Source: CAD feature listing. Evaluate the final solid. Frame: model axes, mm. A direction names the side the tool comes from. Give positions to 0.01 mm unless a question says otherwise; leave off trailing zeros. Loops run counter-clockwise (first coordinate to the right, second up) from the corner with the lowest first, then second, coordinate; pieces in that order, holes last.
```python
from build123d import *

# Parameters (mm, degrees)
F0_R     = 25
F1_DEPTH = 6
F2_R     = 21.4280280098
F3_DEPTH = 3
F4_SIZE  = 5
F6_R     = 21.8410066176
F7_DEPTH = 4
F8_R     = 21.2290439381
F9_DEPTH = 25


# Not quite as in the source:
# - a fillet or chamfer that OpenCascade refuses, or shapes differently, is made with other operations: its cross-section is extruded or revolved along the edge and cut away or added


with BuildPart() as f1:
    # F0 (on Top) → F1 (new body)
    with BuildSketch(Plane.XY):
        Circle(F0_R)
    extrude(amount=F1_DEPTH)

    # F2 (on face) → F3 (join)
    with BuildSketch(Plane.XY.offset(6)):
        Circle(F2_R)
    extrude(amount=-F3_DEPTH)

    # F4
    f4_edges = [f1.edges().sort_by_distance(p)[0] for p in [
        (-25, 0, 6),
    ]]
    chamfer(f4_edges, length=F4_SIZE)

    # F5: fillet of radius 5 on 3 edges, made by hand

    # F5_s1 → F5_t2 (revolve, cut)
    with BuildSketch(Plane.XZ):
        with BuildLine():
            ThreePointArc((25, 0), (24.5002551285, 1.2451619378), (23.687395822, 2.312604178))
            Line((23.687395822, 2.312604178), (25, 1))
            Line((25, 1), (25, 0))
        make_face()
    revolve(axis=Axis((0, 0, 1), (0, 0, 1)), mode=Mode.SUBTRACT)

    # F5_s3 → F5_t4 (revolve, cut)
    with BuildSketch(Plane.XZ):
        with BuildLine():
            ThreePointArc((21.4644660941, 4.5355339059), (19.84234935, 5.6193976626), (17.9289321881, 6))
            Line((17.9289321881, 6), (20, 6))
            Line((20, 6), (21.4644660941, 4.5355339059))
        make_face()
    revolve(axis=Axis((0, 0, 6), (0, 0, 1)), mode=Mode.SUBTRACT)

    # F6 (on face) → F7 (join)
    with BuildSketch(Plane(origin=(0, 0, 0), x_dir=(1, 0, 0), z_dir=(0, 0, -1))):
        Circle(F6_R)
    extrude(amount=-F7_DEPTH)

    # F8 (on face) → F9 (join)
    with BuildSketch(Plane(origin=(0, 0, 0), x_dir=(1, 0, 0), z_dir=(0, 0, -1))):
        Circle(F8_R)
    extrude(amount=F9_DEPTH)


solid = f1.part
```
(1) Ray query, line 1 along Z through (x, y) = (-10.5, -15); line 2 along Y through (x, z) = (0.5, -8.5); line 3 along Y through (x, z) = (18.5, -6). Return the intervals inside material, ascending.
A:
line 1: z = -25 to 5.99
line 2: y = -21.22 to 21.22
line 3: y = -10.41 to 10.41
(2) Reachability of faces 1 (the flat face through (0, 0, -25)), 2 (the flat face through (-11.2, -18.4, 0)) from +Z, -Z, +X, -X, +Y, -Y: full face, straight path, thin tool, end or side. Return the list, or none.
A:
face 1: -Z, +X, -X, +Y, -Y
face 2: -Z
(3) Section C-C, the plane z = -1. Return the cut outline in (x, y), then the cut area to 3 significant figures.
A:
outline: circle Ø42.46 at (0, 0)
area: 1,420 mm2
(4) First-contact query: pin 1 (12 mm diameter, centred on x = -17.5, z = -18, fed in from -Y); pin 2 (1 mm diameter, centred on y = 1.5, z = -6, fed in from -X); pin 3 (12 mm diameter, centred on y = -17, z = -11, fed in from +X). Flat tips, straight axial feed; report the tip coordinate or a pass-through.
A:
pin 1: stops at y = -17.84
pin 2: stops at x = -21.21
pin 3: stops at x = 18.16
(5) Section A-A, the plane x = 0. Return the cut outline in (y, z).
A:
outline: (-25, 0) - (-21.23, 0) - (-21.23, -25) - (21.23, -25) - (21.23, 0) - (25, 0) arc R5 ccw to (23.69, 2.31) - (21.46, 4.54) arc R5 ccw to (17.93, 6) - (-17.93, 6) arc R5 ccw to (-21.46, 4.54) - (-23.69, 2.31) arc R5 ccw to start
